Input: part model. Units: mm. Frame: model coordinates. A direction names the side the tool comes from. Round coordinates to 2 decimals unless told otherwise and drop trailing zeros. Order: outer loops, then holes, each group sorted by start corner. A loop starts at its lowest first (then second) coordinate and runs counter-clockwise, first axis right, second up.
Item 1: Line query: L1, parallel to X at y = -21.5, z = 3; L2, parallel to X at y = -6.5, z = 4; L3, parallel to Z at x = -3.5, y = -21.5. Output: solid intervals per line, ascending.
Item 2: Cut plane D-D on y = -19.75. Output: boundary loops of the cut face in (x, z).
Item 3: Mould query, pull axis Y, two halves, no side actions, for faces 4 (the cylindrical face through (4.73, -3.05, 5.27)), 5 (the cylindrical face through (-0.382, -25.038, 3.219)), 6 (the cylindrical face through (5.07, -0.96, 5.27)). Classes: released by +Y, released by -Y, zero draft, split by the parting line, or undercut.
Item 4: Reachability of faces 1 (the flat face through (1, -6.858, 1)), 2 (the flat face through (-1, -6.858, 3)), 3 (the flat face through (-7.62, -22, 3)) from +Z, -Z, +X, -X, +Y, -Y: full face, straight path, thin tool, end or side. Return the list, or none.
Item 5: Cut plane B-B on z = 3.75. Output: boundary loops of the cut face in (x, y) (3 decimals), then the cut area to 3 significant figures.
Item 6: Cut plane A-A on y = -13.97. Output: boundary loops of the cut face in (x, z) (3 decimals), then the cut area to 3 significant figures.
Item 7: Cut plane C-C on x = 3. Output: boundary loops of the cut face in (y, z).
Item 8: First-contact query: pin 1 (2.5 mm diameter, centred on y = -22.5, z = 3, fed in from +X); pin 2 (2.5 mm diameter, centred on x = 1.5, z = 5.5, fed in from -Y); pin 3 (2.5 mm diameter, centred on y = -4.5, z = 3.5, fed in from +X). Flat tips, straight axial feed; report the tip coordinate or a pass-through.
```python
from build123d import *

# Parameters (mm, degrees)
F0_R            = 1.27
F1_DEPTH        = 6.35
F3_W            = 6.858
F3_H            = 2.1082
F4_DEPTH        = 7.62
F5_R            = 1.27
F6_W            = 6.35
F6_H            = 2.2097155452
F7_DEPTH        = 6.35
F9_D            = 2.54
F9_CBORE_D      = 2.54
F9_CBORE_DEPTH  = 6.35
F11_D           = 2.54
F11_CBORE_D     = 2.54
F11_CBORE_DEPTH = 6.35
F12_T1_DEPTH    = 21.1836
F12_T3_DEPTH    = 21.1582


# Not quite as in the source:
# - a fillet or chamfer that OpenCascade refuses, or shapes differently, is made with other operations: its cross-section is extruded or revolved along the edge and cut away or added


with BuildPart() as f1:
    # F0 (on Top) → F1 (new body)
    with BuildSketch(Plane.XY):
        Polygon((6.35, 0), (0, 0), (-8.89, 0), (-8.89, -6.858), (-8.89, -25.4), (0, -25.4), (0, -6.858), (6.35, -6.858), align=None)
        with Locations((3.5186004825, -3.429)):
            Circle(F0_R, mode=Mode.SUBTRACT)
    extrude(amount=F1_DEPTH)

    # F3 (on face) → F4 (cut)
    with BuildSketch(Plane.YZ.offset(6.35)):
        with Locations((-3.429, 3.1623)):
            Rectangle(F3_W, F3_H)
    extrude(amount=-F4_DEPTH, mode=Mode.SUBTRACT)

    # F5
    f5_edges = [f1.edges().sort_by_distance(p)[0] for p in [
        (0, -25.4, 3.175),
        (-8.89, -25.4, 3.175),
        (-8.89, 0, 3.175),
    ]]
    fillet(f5_edges, radius=F5_R)

    # F6 (on face) → F7 (cut)
    with BuildSketch(Plane.XZ.offset(25.4)):
        with Locations((-4.445, 3.1112665311)):
            Rectangle(F6_W, F6_H)
    extrude(amount=-F7_DEPTH, mode=Mode.SUBTRACT)

    # F9 (through all)
    with Locations(Plane.XY.offset(6.35)):
        with Locations((-4.5120492578, -23.6996337771)):
            CounterBoreHole(F9_D / 2, F9_CBORE_D / 2, F9_CBORE_DEPTH)

    # F11 (through all)
    with Locations(Plane.XY.offset(6.35)):
        with Locations((-4.445, -13.97)):
            CounterBoreHole(F11_D / 2, F11_CBORE_D / 2, F11_CBORE_DEPTH)

    # F12: fillet of radius 3.81 on 4 edges, made by hand

    # F12_s2 → F12_t1 (cut)
    with BuildSketch(Plane.XY.offset(-5.3086)):
        with BuildLine():
            ThreePointArc((6.35, -3.048), (5.2340768363, -5.7420768363), (2.54, -6.858))
            Line((2.54, -6.858), (6.35, -6.858))
            Line((6.35, -6.858), (6.35, -3.048))
        make_face()
        with BuildLine():
            ThreePointArc((2.54, 0), (5.2340768363, -1.1159231637), (6.35, -3.81))
            Line((6.35, -3.81), (6.35, 0))
            Line((6.35, 0), (2.54, 0))
        make_face()
    extrude(amount=F12_T1_DEPTH, mode=Mode.SUBTRACT)

    # F12_s4 → F12_t3 (cut)
    with BuildSketch(Plane.XY.offset(-9.525)):
        with BuildLine():
            ThreePointArc((6.35, -3.048), (5.2340768363, -5.7420768363), (2.54, -6.858))
            Line((2.54, -6.858), (6.35, -6.858))
            Line((6.35, -6.858), (6.35, -3.048))
        make_face()
        with BuildLine():
            ThreePointArc((2.54, 0), (5.2340768363, -1.1159231637), (6.35, -3.81))
            Line((6.35, -3.81), (6.35, 0))
            Line((6.35, 0), (2.54, 0))
        make_face()
    extrude(amount=F12_T3_DEPTH, mode=Mode.SUBTRACT)


solid = f1.part
```
From the geometry:
1. L1: x = -8.89 to -7.62, -1.27 to 0
1. L2: x = -8.89 to -1.27
1. L3: z = 0 to 2.01, 4.22 to 6.35
2. outline: (-8.89, 0) - (0, 0) - (0, 6.35) - (-8.89, 6.35) - close; hole (-7.62, 2.01) - (-1.27, 2.01) - (-1.27, 4.22) - (-7.62, 4.22) - close
3. face 4: undercut
3. face 5: released by -Y
3. face 6: released by +Y
4. face 1: +Z, -Z, +X, -Y
4. face 2: +X, +Y
4. face 3: -Y
5. outline: (-8.89, -24.13) arc R1.27 ccw to (-7.62, -25.4) - (-7.62, -19.05) - (-1.27, -19.05) - (-1.27, -25.4) arc R1.27 ccw to (0, -24.13) - (0, -6.858) - (-1.27, -6.858) - (-1.27, 0) - (-7.62, 0) arc R1.27 ccw to (-8.89, -1.27) - close; hole circle Ø2.54 at (-4.445, -13.97)
5. area: 171 mm2
6. outline: (-8.89, 0) - (-5.715, 0) - (-5.715, 6.35) - (-8.89, 6.35) - close; (-3.175, 0) - (0, 0) - (0, 6.35) - (-3.175, 6.35) - close
6. area: 40.3 mm2
7. outline: (-6.83, 0) - (-4.59, 0) - (-4.59, 2.11) - (-6.83, 2.11) - close; (-6.83, 4.22) - (-4.59, 4.22) - (-4.59, 6.35) - (-6.83, 6.35) - close; (-2.27, 0) - (-0.03, 0) - (-0.03, 2.11) - (-2.27, 2.11) - close; (-2.27, 4.22) - (-0.03, 4.22) - (-0.03, 6.35) - (-2.27, 6.35) - close
8. pin 1: stops at x = 0
8. pin 2: stops at y = -6.86
8. pin 3: stops at x = 6.33
